Can you work these out from the model? Positions are in its coordinate system, mm. A direction names the side the tool comes from. Give positions to 0.01 mm unless a question says otherwise; leave off trailing zeros. Order: outer loops, then holes, each group sorted by start corner. A loop starts at its lowest first (then second) coordinate and runs counter-clockwise, first axis right, second up. Notation, with made-up numbers: (8.5, 83) - (34.5, 83) arc R20 cw to (34.5, 115) - close; hole circle Ø9 at (83.5, 62). An arc over 180 degrees is marked (long way). Answer as a JSON object with one key per item and string values.
```python
from build123d import *


with BuildPart() as f1:
    # F0 (on Front) → F1 (revolve)
    with BuildSketch(Plane.XZ):
        Polygon((-7.087499, 8), (-7.087499, 0), (-3.487499, 0), (-3.487499, 8), (0, 8), (0, 10), (-3.487499, 10), (-3.487499, 18), (0, 18), (0, 20), (-3.487499, 20), (-3.487499, 24.6), (-3.187499, 24.6), (-3.433158, 24.772198), (-3.433158, 30.150307), (-3.133158, 30.150307), (-3.433158, 30.428462), (-3.433158, 37.6), (-7.087499, 37.6), (-7.141841, 30.428462), (-7.387499, 30.150307), (-7.141841, 30.150307), (-7.141841, 24.772198), (-7.387499, 24.6), (-7.087499, 24.6), (-7.087499, 20), (-10.574999, 20), (-10.574999, 17.674999), (-7.087499, 17.674999), (-7.087499, 10), (-10.574999, 10), (-10.574999, 8), align=None)
    revolve(axis=Axis((0, 0, 19), (0, 0, 1)))


solid = f1.part
```
Q1. Which directions (+Z, -Z, +X, -X, +Y, -Y) give clear straight access to the entire face, cutting with the end or side of a thin tool? Please do faces 4 (the face through (-7, 2, 8)), 5 (the face through (1.67, -3.25, 0)), 6 (the face through (-6.597, 2.735, 27.424)).
Recorded:
{"face 4": "-Z", "face 5": "-Z, +X, -X, +Y, -Y", "face 6": "none"}
Q2. If we section it at C-C, the plane z = 35.5: Please give me the cut outline in (x, y).
Recorded:
{"outline": "circle Ø14.21 at (0, 0); hole circle Ø6.87 at (0, 0)"}
Q3. If we section it at A-A, the plane y = 9.25: Please give me the cut outline in (x, z) (3 decimals).
Recorded:
{"outline": "(-5.125, 8) - (5.125, 8) - (5.125, 10) - (-5.125, 10) - close; (-5.125, 17.675) - (5.125, 17.675) - (5.125, 20) - (-5.125, 20) - close"}
Q4. If we section it at B-B, the plane z = 26.5: Please give me the cut outline in (x, y).
Recorded:
{"outline": "circle Ø14.28 at (0, 0); hole circle Ø6.87 at (0, 0)"}
Q5. I need wall thicknesses on L1, parallel to X at y = 0, z = 26.65; L2, parallel to Z at x = 3.75, y = 9.75 (3 decimals). Which ranges of each line are inside material? Lowest first, please.
Recorded:
{"L1": "x = -7.14 to -3.43, 3.43 to 7.14", "L2": "z = 8 to 10, 17.675 to 20"}
Q6. We'd pull the mould along Y, two halves only. Please class faces 1 (the face through (-10.087, -3.176, 8.986)), 2 (the face through (3, -2, 37.6)), 3 (the face through (-3.275, -1.031, 34.064)): released by +Y, released by -Y, zero draft, split by the parting line, or undercut.
Recorded:
{"face 1": "split by the parting line", "face 2": "zero draft", "face 3": "undercut"}
Q7. I'm going to push flat-ended pins straight in: pin 1 Ø8 at (x, z) = (-4.5, 33) entering from -Y; pin 2 Ø1 at (x, z) = (-1, 28.5) entering from +Y; pin 3 Ø6.5 at (x, y) = (0, 0) entering from +Z. Where does each tip first touch, or does it pass through?
Recorded:
{"pin 1": "stops at y = -7.19", "pin 2": "stops at y = 7.12", "pin 3": "stops at z = 30.26"}
